```python
from build123d import *

# Parameters (mm, degrees)
F0_W     = 180
F0_H     = 150
F1_DEPTH = 199
F2_R     = 20
F3_R     = 20
F4_W     = 387.1927191635
F4_H     = 130
F5_DEPTH = 190
F7_DEPTH = 160
F8_R     = 10
F9_DEPTH = 264.3
F10_R    = 2
F11_R    = 5


with BuildPart() as f1:
    # F0 (on Front) → F1 (new body)
    with BuildSketch(Plane.XZ):
        with Locations((-49.0434786677, 4.1188420764)):
            Rectangle(F0_W, F0_H)
    extrude(amount=F1_DEPTH)

    # F2
    f2_edges = [f1.edges().sort_by_distance(p)[0] for p in [
        (-49.043479, -199, 79.118842),
    ]]
    fillet(f2_edges, radius=F2_R)

    # F3
    f3_edges = [f1.edges().sort_by_distance(p)[0] for p in [
        (-139.043479, -89.5, 79.118842),
    ]]
    fillet(f3_edges, radius=F3_R)

    # F4 (on Front) → F5 (cut)
    with BuildSketch(Plane.XZ):
        with Locations((64.552880914, 4.1188420764)):
            Rectangle(F4_W, F4_H)
    extrude(amount=F5_DEPTH, mode=Mode.SUBTRACT)

    # F6 (on face) → F7 (cut)
    with BuildSketch(Plane.YZ.offset(40.9565213323)):
        Polygon((-133.5333704529, 74.1188420764), (-141.0166852265, 79.1188420764), (-161.0166852265, 79.1188420764), (-168.5, 74.1188420764), (-161.0166852265, 69.1188420764), (-141.0166852265, 69.1188420764), align=None)
        Polygon((-84.9833147735, 79.1188420764), (-104.9833147735, 79.1188420764), (-112.4666295471, 74.1188420764), (-104.9833147735, 69.1188420764), (-84.9833147735, 69.1188420764), (-77.5, 74.1188420764), align=None)
        Polygon((-28.9833147735, 79.1188420764), (-48.9833147735, 79.1188420764), (-56.4666295471, 74.1188420764), (-48.9833147735, 69.1188420764), (-28.9833147735, 69.1188420764), (-21.5, 74.1188420764), align=None)
    extrude(amount=-F7_DEPTH, mode=Mode.SUBTRACT)

    # F8 (on Front) → F9 (cut)
    with BuildSketch(Plane.XZ):
        with Locations((-89.0434786677, -40.8811579236)):
            Circle(F8_R)
    extrude(amount=F9_DEPTH, mode=Mode.SUBTRACT)

    # F10
    f10_edges = [f1.edges().sort_by_distance(p)[0] for p in [
        (40.956521, -199, -5.881158),
        (40.956521, -193.142136, 73.260978),
        (40.956521, -123, 79.118842),
        (40.956521, -66.983315, 79.118842),
        (40.956521, -14.491657, 79.118842),
    ]]
    fillet(f10_edges, radius=F10_R)

    # F11
    f11_edges = [f1.edges().sort_by_distance(p)[0] for p in [
        (-99.043479, -199, -40.881158),
    ]]
    fillet(f11_edges, radius=F11_R)

    # F12: F1 across plane


with BuildPart() as f1_1:
    add(f1.part)
    add(f1.part.mirror(Plane.XZ))


solid = f1_1.part
```
The listing builds one solid part. Answer for the finished solid, in the listing's coordinates (mm). A direction names the side the tool comes from. Give positions to 0.01 mm unless a question says otherwise; leave off trailing zeros. Order: outer loops, then holes, each group sorted by start corner. A loop starts at its lowest first (then second) coordinate and runs counter-clockwise, first axis right, second up. Notation, with made-up numbers: (-27, -36.75) - (-16, -36.75) arc R27 ccw to (-16, -2.75) - close; hole circle Ø1 at (-0.75, 66.25). An arc over 180 degrees is marked (long way). Answer in a Markdown table with one row per item. Add a question column.
Q1. Find the intervals of material crossed by line 1 along Y through (x, z) = (32.5, -53.5); line 2 along Z through (x, y) = (12, 8); line 3 along Z through (x, y) = (-10.5, -161.5), in increasing order. Write a range as [from, to].
Q2. For a pull along Y with two mould halves and no side action, classify faces 1 (the flat face through (40.957, -123, 73)), 2 (the flat face through (-129.043, -3, 3)), 3 (the cylindrical face through (-38.9, 193, 73.4)) as released by +Y, released by -Y, zero draft, split by the parting line, or undercut.
Q3. Which of the six approach directions +Z, -Z, +X, -X, +Y, -Y give full straight-line access (tool end or side, diameter ignored) to faces 4 (the flat face through (-119.043, -39, 74)), 5 (the cylindrical face through (-79.8, 192, -44.7))?
Q4. The part is cut by section C-C (x = -68.5). Give the number of separate pieces and of enclosed holes in the cut face, then the cut area to 3 significant figures.
Q5. Given P1, Ø3, axis at y = -93.5, z = 74.5, coming from the +X side; P2, Ø3, axis at y = -13.5, z = 3, coming from the +X side, each flat-ended and moving along its own axis, determine where each tip first touches the part or whether it passes through.
Q6. The part is cut by section A-A (y = -61). Determine the outline of the cut face in (x, z).
Q7. The part is cut by section B-B (z = 16.5). Determine the outline of the cut face in (x, y).
Determined:
| question | item | result |
|---|---|---|
| 1 | line 1 | y = [-199, -190], [190, 199] |
| 1 | line 2 | z = [-70.88, -60.88], [69.12, 79.12] |
| 1 | line 3 | z = [-70.88, -60.88], [69.12, 69.44], [78.8, 79.12] |
| 2 | face 1 | zero draft |
| 2 | face 2 | undercut |
| 2 | face 3 | released by +Y |
| 3 | face 4 | +X |
| 3 | face 5 | +Y, -Y |
| 4 | separate pieces | 6 |
| 4 | enclosed holes | 0 |
| 4 | area | 8,480 mm² |
| 5 | P1 | stops at x = -119.04 |
| 5 | P2 | stops at x = -129.04 |
| 6 | outline | (-139.04, -70.88) - (40.96, -70.88) - (40.96, -60.88) - (-129.04, -60.88) - (-129.04, 69.12) - (40.96, 69.12) - (40.96, 77.12) arc R2 ccw to (38.96, 79.12) - (-119.04, 79.12) arc R20 ccw to (-139.04, 59.12) - close |
| 7 | outline | (-139.04, -179) arc R20 ccw to (-119.04, -199) - (38.96, -199) arc R2 ccw to (40.96, -197) - (40.96, -190) - (-129.04, -190) - (-129.04, 190) - (40.96, 190) - (40.96, 197) arc R2 ccw to (38.96, 199) - (-119.04, 199) arc R20 ccw to (-139.04, 179) - close |
